Verification items for the finished model (mm, model axes). Face numbers are marked on the shaded views. Coordinates: 2 decimals unless noted, no trailing zeros. Order: outer loops, then holes, each group sorted by start corner. A loop starts at its lowest first (then second) coordinate and runs counter-clockwise, first axis right, second up. Notation, with made-up numbers: M 70.5,-39 L 114.5,-39 A15 cw 114.5,-16 Z; hole C -2,19 d7. An arc over 180 degrees is marked long. Return JSON: item names as keys, results as strings. Group by question number.
Q1. Section check A-A, the plane y = -31.8. Enter the section's corners in (x, z), then the cut area to 3 significant figures.
Q2. Thickness scan on probe 1 along Z at (x, y) = (14, -3); probe 2 along Z at (x, y) = (2, -23); probe 3 along Y at (x, z) = (-12.5, -1.75). Record the ranges inside material, lowest first.
Q3. Section check C-C, the plane z = 2. Enter the section's corners in (x, y).
Q4. Mould release check, pull along Z, two halves, no side actions. Record for the marked faces 1, 2 and 3: pulls with the +Z half, pulls with the -Z half, needs draft (parallel to the pull), parting line crosses it, or undercut.
Q5. Section check B-B, the plane x = 8. Enter the section's corners in (y, z).
Q6. Go/stop test with flat-tipped pins: pin 1 Ø3.5 at (x, y) = (10, -14) entering from +Z; pin 2 Ø0.9 at (x, y) = (-6.5, -6.5) entering from +Z; pin 3 Ø0.9 at (x, z) = (8, 1.5) entering from -Y. Record where each tip stops, or that it passes through.
Q7. Section check D-D, the plane y = -23.5. Enter the section's corners in (x, z).
from build123d import *

# Parameters (mm, degrees)
F0_W     = 32
F0_H     = 32
F1_DEPTH = 3
F2_W     = 32
F2_H     = 50
F3_DEPTH = 13
F4_R     = 1.5
F5_DEPTH = 0.1
F6_R     = 1.5
F7_DEPTH = 13.001


with BuildPart() as f1:
    # F0 (on Top) → F1 (new body)
    with BuildSketch(Plane.XY):
        Rectangle(F0_W, F0_H)
    extrude(amount=F1_DEPTH)

    # F2 (on face) → F3 (join)
    with BuildSketch(Plane(origin=(0, 0, 0), x_dir=(1, 0, 0), z_dir=(0, 0, -1))):
        with Locations((0, 9)):
            Rectangle(F2_W, F2_H)
    extrude(amount=F3_DEPTH)

    # F4 (on face) → F5 (cut)
    with BuildSketch(Plane.XY.offset(3)):
        with Locations((14, 14)):
            Circle(F4_R)
        with Locations((14, 10)):
            Circle(F4_R)
        with Locations((14, 6)):
            Circle(F4_R)
        with Locations((14, 2)):
            Circle(F4_R)
        with Locations((14, -2)):
            Circle(F4_R)
        with Locations((14, -6)):
            Circle(F4_R)
        with Locations((14, -10)):
            Circle(F4_R)
        with Locations((14, -14)):
            Circle(F4_R)
        with Locations((10, 14)):
            Circle(F4_R)
        with Locations((10, 10)):
            Circle(F4_R)
        with Locations((10, 6)):
            Circle(F4_R)
        with Locations((10, 2)):
            Circle(F4_R)
        with Locations((10, -2)):
            Circle(F4_R)
        with Locations((10, -6)):
            Circle(F4_R)
        with Locations((10, -10)):
            Circle(F4_R)
        with Locations((10, -14)):
            Circle(F4_R)
        with Locations((6, 14)):
            Circle(F4_R)
        with Locations((6, 10)):
            Circle(F4_R)
        with Locations((6, 6)):
            Circle(F4_R)
        with Locations((6, 2)):
            Circle(F4_R)
        with Locations((6, -2)):
            Circle(F4_R)
        with Locations((6, -6)):
            Circle(F4_R)
        with Locations((6, -10)):
            Circle(F4_R)
        with Locations((6, -14)):
            Circle(F4_R)
        with Locations((2, 14)):
            Circle(F4_R)
        with Locations((2, 10)):
            Circle(F4_R)
        with Locations((2, 6)):
            Circle(F4_R)
        with Locations((2, 2)):
            Circle(F4_R)
        with Locations((2, -2)):
            Circle(F4_R)
        with Locations((2, -6)):
            Circle(F4_R)
        with Locations((2, -10)):
            Circle(F4_R)
        with Locations((2, -14)):
            Circle(F4_R)
        with Locations((-2, 14)):
            Circle(F4_R)
        with Locations((-2, 10)):
            Circle(F4_R)
        with Locations((-2, 6)):
            Circle(F4_R)
        with Locations((-2, 2)):
            Circle(F4_R)
        with Locations((-2, -2)):
            Circle(F4_R)
        with Locations((-2, -6)):
            Circle(F4_R)
        with Locations((-2, -10)):
            Circle(F4_R)
        with Locations((-2, -14)):
            Circle(F4_R)
        with Locations((-6, 14)):
            Circle(F4_R)
        with Locations((-6, 10)):
            Circle(F4_R)
        with Locations((-6, 6)):
            Circle(F4_R)
        with Locations((-6, 2)):
            Circle(F4_R)
        with Locations((-6, -2)):
            Circle(F4_R)
        with Locations((-6, -6)):
            Circle(F4_R)
        with Locations((-6, -10)):
            Circle(F4_R)
        with Locations((-6, -14)):
            Circle(F4_R)
        with Locations((-10, 14)):
            Circle(F4_R)
        with Locations((-10, 10)):
            Circle(F4_R)
        with Locations((-10, 6)):
            Circle(F4_R)
        with Locations((-10, 2)):
            Circle(F4_R)
        with Locations((-10, -2)):
            Circle(F4_R)
        with Locations((-10, -6)):
            Circle(F4_R)
        with Locations((-10, -10)):
            Circle(F4_R)
        with Locations((-10, -14)):
            Circle(F4_R)
        with Locations((-14, 14)):
            Circle(F4_R)
        with Locations((-14, 10)):
            Circle(F4_R)
        with Locations((-14, 6)):
            Circle(F4_R)
        with Locations((-14, 2)):
            Circle(F4_R)
        with Locations((-14, -2)):
            Circle(F4_R)
        with Locations((-14, -6)):
            Circle(F4_R)
        with Locations((-14, -10)):
            Circle(F4_R)
        with Locations((-14, -14)):
            Circle(F4_R)
    extrude(amount=-F5_DEPTH, mode=Mode.SUBTRACT)

    # F6 (on face) → F7 (cut, through all)
    with BuildSketch(Plane.XY):
        with Locations((-13.8, -31.8)):
            Circle(F6_R)
        with Locations((13.8, -31.8)):
            Circle(F6_R)
    extrude(amount=-F7_DEPTH, mode=Mode.SUBTRACT)


solid = f1.part
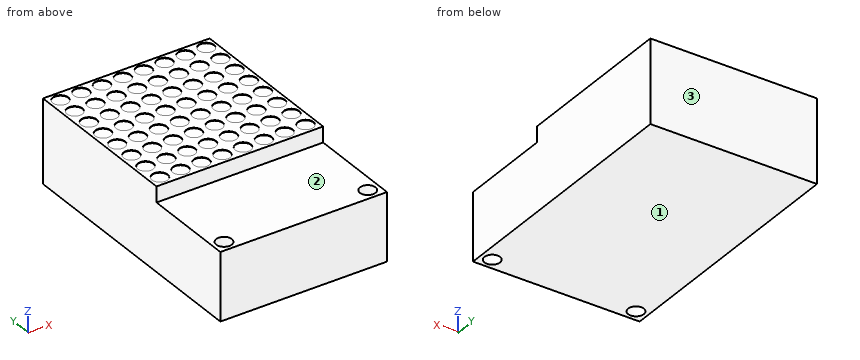
Numbers:
{
 "1": {"outline": "M -16,-13 L -15.3,-13 L -15.3,0 L -16,0 Z; M -12.3,-13 L 12.3,-13 L 12.3,0 L -12.3,0 Z; M 15.3,-13 L 16,-13 L 16,0 L 15.3,0 Z", "area": "338 mm2"},
 "2": {"probe 1": "z = -13 to 2.9", "probe 2": "z = -13 to 0", "probe 3": "y = -34 to -32.55, -31.05 to 16"},
 "3": {"outline": "M -16,-16 L 16,-16 L 16,16 L -16,16 Z"},
 "4": {"face 1": "pulls with the -Z half", "face 2": "pulls with the +Z half", "face 3": "needs draft"},
 "5": {"outline": "M -34,-13 L 16,-13 L 16,3 L -16,3 L -16,0 L -34,0 Z"},
 "6": {"pin 1": "stops at z = 3", "pin 2": "stops at z = 2.9", "pin 3": "stops at y = -16"},
 "7": {"outline": "M -16,-13 L 16,-13 L 16,0 L -16,0 Z"}
}
